from build123d import *

# Parameters (mm, degrees)
F0_R     = 3
F1_DEPTH = 5
F2_SIZE  = 0.5


with BuildPart() as f1:
    # F0 (on Front) → F1 (new body)
    with BuildSketch(Plane.XZ):
        Polygon((2.886751, 5), (-2.886751, 5), (-5.773503, 0), (-2.886751, -5), (2.886751, -5), (5.773503, 0), align=None)
        Circle(F0_R, mode=Mode.SUBTRACT)
    extrude(amount=F1_DEPTH)

    # F2
    f2_edges = [f1.edges().sort_by_distance(p)[0] for p in [
        (4.330127, -5, 2.5),
        (0, -5, 5),
        (-4.330127, -5, 2.5),
        (-4.330127, -5, -2.5),
        (0, -5, -5),
        (4.330127, -5, -2.5),
        (-3, -5, 0),
        (4.330127, 0, 2.5),
        (0, 0, 5),
        (-4.330127, 0, 2.5),
        (-4.330127, 0, -2.5),
        (0, 0, -5),
        (4.330127, 0, -2.5),
        (-3, 0, 0),
    ]]
    chamfer(f2_edges, length=F2_SIZE)


solid = f1.part
Could you check a few things on this model? Use its own coordinates, in mm. Give positions to 0.01 mm unless a question says otherwise; leave off trailing zeros. Loops run counter-clockwise (first coordinate to the right, second up) from the corner with the lowest first, then second, coordinate; pieces in that order, holes last. Notation, with made-up numbers: M 30.25,11.25 L 77.25,11.25 A7 cw 77.25,23.25 Z; hole C 75,65.5 d11. An arc over 180 degrees is marked long. Answer as a JSON object with one key per item and string values.
Q1. For P1, Ø1.5, axis at y = -1.5, z = 0.5, coming from the +X side; P2, Ø1, axis at x = -3, y = -4, coming from the +Z side, each with a flat end and sliding along its axis, tell me the tip position at first contact or that it passes through.
Values found:
{"P1": "stops at x = 5.77", "P2": "stops at z = 5"}
Q2. Suppose I cut it at D-D, the plane x = -4.5. List the corners of the cut face in (y, z) for me.
Values found:
{"outline": "M -5,-1.21 L -4.5,-2.21 L -0.5,-2.21 L 0,-1.21 L 0,1.21 L -0.5,2.21 L -4.5,2.21 L -5,1.21 Z"}
Q3. Suppose I cut it at A-A, the plane x = 0. List the corners of the cut face in (y, z) for me.
Values found:
{"outline": "M -5,-4.5 L -4.5,-5 L -0.5,-5 L 0,-4.5 L 0,-3.5 L -0.5,-3 L -4.5,-3 L -5,-3.5 Z; M -5,3.5 L -4.5,3 L -0.5,3 L 0,3.5 L 0,4.5 L -0.5,5 L -4.5,5 L -5,4.5 Z"}
Q4. If I drill on probe 1 along Z at (x, y) = (0, -2.5); probe 2 along X at (y, z) = (-3, 1); probe 3 along Z at (x, y) = (-1.25, -1.9), over which ranges is the centre line in solid material (lowest first)? Write a range as [from, to].
Values found:
{"probe 1": "z = [-5, -3], [3, 5]", "probe 2": "x = [-5.2, -2.83], [2.83, 5.2]", "probe 3": "z = [-5, -2.73], [2.73, 5]"}
Q5. Suppose I cut it at C-C, the plane z = 4. List the corners of the cut face in (x, y) for me.
Values found:
{"outline": "M -3.46,-4.5 L -2.89,-5 L 2.89,-5 L 3.46,-4.5 L 3.46,-0.5 L 2.89,0 L -2.89,0 L -3.46,-0.5 Z"}
Q6. Suppose I cut it at B-B, the plane y = -2.3. List the corners of the cut face in (x, z) for me.
Values found:
{"outline": "M -5.77,0 L -2.89,-5 L 2.89,-5 L 5.77,0 L 2.89,5 L -2.89,5 Z; hole C 0,0 d6"}
Q7. If we mould it in two halves opening along X, with no side actions, what happens to faces 1 (the cylindrical face through (-3, -2, 0)), 2 (the flat face through (-4.09, -0.247, 2.408)), 3 (the flat face through (4.31, -2.472, -2.535))? For each: pulls with the +X half, pulls with the -X half, needs draft (parallel to the pull), parting line crosses it, or undercut.
Values found:
{"face 1": "undercut", "face 2": "pulls with the -X half", "face 3": "pulls with the +X half"}
